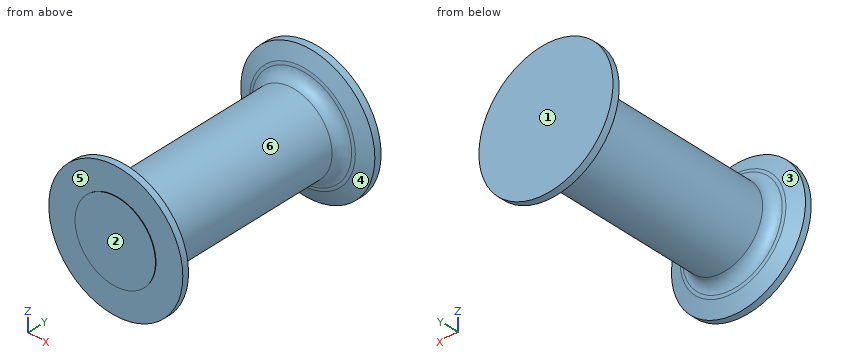
from build123d import *

# Parameters (mm, degrees)
F0_R     = 19.05
F1_DEPTH = 101.6
F2_R     = 31.75
F3_DEPTH = 6.35
F5_START = 95.25
F4_R     = 31.75
F5_DEPTH = 6.096
F6_SIZE  = 2.54
F8_R     = 5.08
F9_R     = 5.08


# Not quite as in the source:
# - a fillet or chamfer that OpenCascade refuses, or shapes differently, is made with other operations: its cross-section is extruded or revolved along the edge and cut away or added


with BuildPart() as f1:
    # F0 (on Front) → F1 (new body)
    with BuildSketch(Plane.XZ):
        Circle(F0_R)
    extrude(amount=F1_DEPTH)

    # F2 (on Front) → F3 (join)
    with BuildSketch(Plane.XZ):
        Circle(F2_R)
    extrude(amount=F3_DEPTH)

    # F4 (on Front) → F5 (join)
    with BuildSketch(Plane.XZ.offset(F5_START)):
        Circle(F4_R)
    extrude(amount=F5_DEPTH)

    # F6
    f6_edges = [f1.edges().sort_by_distance(p)[0] for p in [
        (-31.75, -6.35, 0),
        (-31.75, -95.25, 0),
    ]]
    chamfer(f6_edges, length=F6_SIZE)

    # F7: chamfer of 5.08 on 2 edges, made by hand

    # F7_s1 → F7_t2 (revolve, cut)
    with BuildSketch(Plane.XY):
        Polygon((24.13, -95.25), (32.8021024484, -98.8421024484), (29.21, -95.25), align=None)
    revolve(axis=Axis((0, -95.25, 0), (0, -1, 0)), mode=Mode.SUBTRACT)

    # F7_s3 → F7_t4 (revolve, cut)
    with BuildSketch(Plane.XY):
        Polygon((32.8021024484, -2.7578975516), (24.13, -6.35), (29.21, -6.35), align=None)
    revolve(axis=Axis((0, -6.35, 0), (0, -1, 0)), mode=Mode.SUBTRACT)

    # F8
    f8_edges = [f1.edges().sort_by_distance(p)[0] for p in [
        (-24.13, -6.35, 0),
        (-24.13, -95.25, 0),
    ]]
    fillet(f8_edges, radius=F8_R)

    # F9
    f9_edges = [f1.edges().sort_by_distance(p)[0] for p in [
        (-19.05, -95.25, 0),
        (-19.05, -6.35, 0),
    ]]
    fillet(f9_edges, radius=F9_R)


solid = f1.part
Part model, mm, in its own coordinate system. Face numbers are marked on the shaded views. A direction names the side the tool comes from. Coordinates: 2 decimals unless noted, no trailing zeros. Loops run counter-clockwise (first coordinate to the right, second up) from the corner with the lowest first, then second, coordinate; pieces in that order, holes last. Notation, with made-up numbers: (87.25, -30) -> (102.25, -30) arc R31 ccw to (102.25, -4) -> close; hole circle Ø4 at (7.5, 33). An arc over 180 degrees is marked (long way). Use a Markdown table: item, result. Add a question column.
Item 1: Probe probe 1 along Y at (x, z) = (18.5, 17); probe 2 along Y at (x, z) = (1, -26); probe 3 along Z at (x, y) = (0, -57). List the from-to ranges inside material, lowest first.
Item 2: Pull direction Y, two halves, no side cores. Call the marked faces 1, 2, 3 and 4: +Y half, -Y half, draft (parallel to the pull), parting line (faces both ways), or undercut.
Item 3: Flat gauge pins, fed straight in: P1, Ø12, axis at x = -14, z = -23.5, coming from the +Y side; P2, Ø6, axis at y = -20.5, z = -17, coming from the +X side; P3, Ø4, axis at y = -59, z = -18.5, coming from the -X side; P4, Ø2, axis at x = -8, y = -39.5, coming from the -Z side. Where does each tip first touch, or does it go through?
Item 4: Band-saw the part on A-A on y = -28.5. Write the cut outline in (x, z).
Item 5: Which spindle directions (+Z, -Z, +X, -X, +Y, -Y) get a long thin tool onto all of the face, cutting with end or side? Do the marked faces 5 and 6. Say none if no direction does.
Geometry says:
| question | item | result |
|---|---|---|
| 1 | probe 1 | -101.35 to -95.66, -5.94 to 0 |
| 1 | probe 2 | -101.35 to -96.03, -5.57 to 0 |
| 1 | probe 3 | -19.05 to 19.05 |
| 2 | face 1 | +Y half |
| 2 | face 2 | -Y half |
| 2 | face 3 | undercut |
| 2 | face 4 | undercut |
| 3 | P1 | y = 0 |
| 3 | P2 | x = 12.92 |
| 3 | P3 | x = -9.52 |
| 3 | P4 | z = -17.72 |
| 4 | outline | circle Ø38.1 at (0, 0) |
| 5 | face 5 | -Y |
| 5 | face 6 | none |
